Geometry: see drawing. Coordinates: mm, zero at the bounding-box minimum. A direction names the side the tool comes from. Give positions to 0.01 mm unless a question says otherwise; leave off trailing zeros. Order: outer loops, then holes, each group sorted by start corner. A loop starts at its lowest first (then second) coordinate and runs counter-clockwise, first axis right, second up. Notation, with made-up numbers: (39, -30) - (56, -30) arc R21 cw to (56, -21) - close; hole circle Ø8 at (55.5, 70.25). An arc over 180 degrees is marked (long way). Write each question's results on one line, items separated by ' | '. Start each with the question number.
Item 1: Contact query for a flat-ended pin moving along its axis: pin 1 Ø6 at (x, y) = (16.51, 56.34) entering from +Z. Output: stop coordinate, or through.
Item 2: Line query: line 1 along X through (y, z) = (55, 5.75); line 2 along Z through (x, y) = (3.5, 8). Output: solid intervals per line, ascending.
Item 3: Section C-C on y = 32.5. Output: boundary loops of the cut face in (x, z), and give its area (3 significant figures).
Item 4: Set-up query: the marked faces 1 and 2. Return all of +Z, -Z, +X, -X, +Y, -Y with unobstructed straight access to the full face (end or side cutting, diameter ignored); none if empty.
Item 5: Section A-A on z = 9.5. Output: boundary loops of the cut face in (x, y).
Item 6: Section B-B on y = 55. Output: boundary loops of the cut face in (x, z) (1 decimal).
Item 7: Section D-D on x = 10. Output: boundary loops of the cut face in (y, z).
Item 8: Mould query, pull axis X, two halves, no side actions, for the marked faces 3, 4 and 5. Classes: released by +X, released by -X, zero draft, split by the parting line, or undercut.
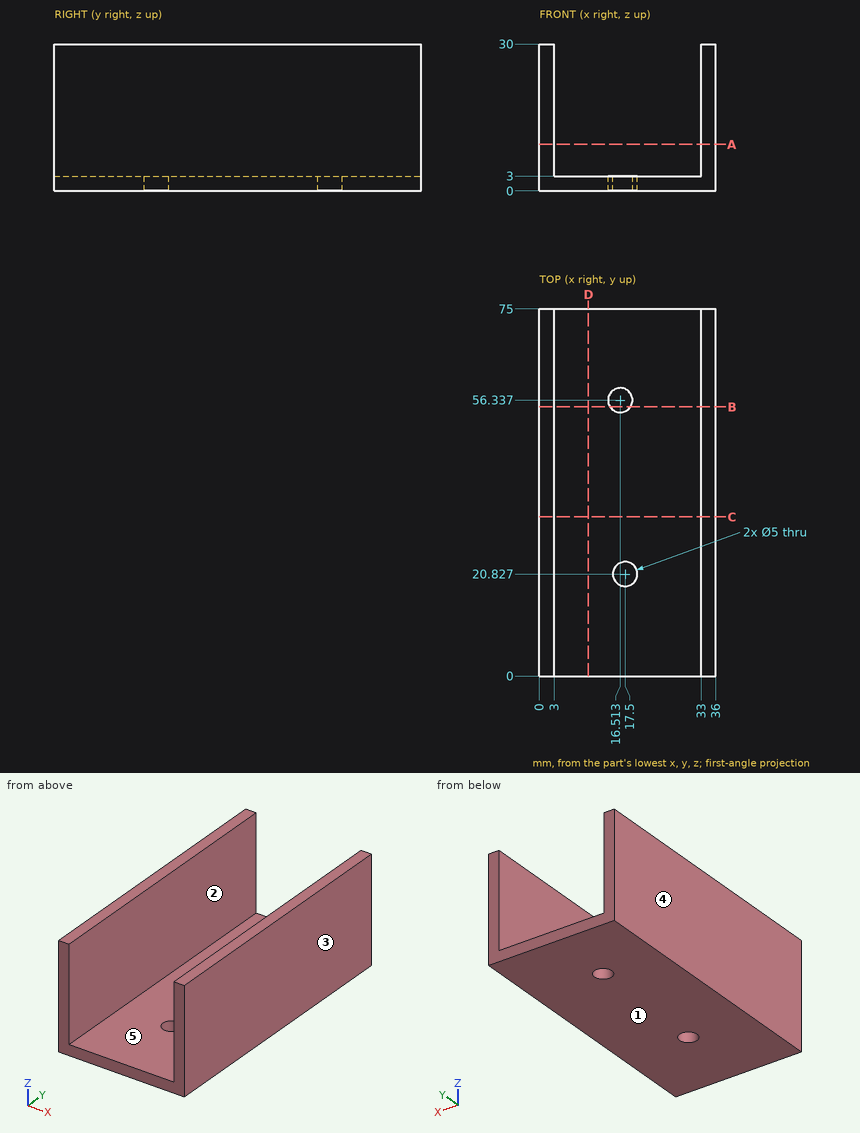
Evaluation:
1) pin 1: stops at z = 3
2) line 1: x = 0 to 3, 33 to 36 | line 2: z = 0 to 3
3) outline: (0, 0) - (36, 0) - (36, 30) - (33, 30) - (33, 3) - (3, 3) - (3, 30) - (0, 30) - close | area: 270 mm^2
4) face 1: -Z, +X, -X, +Y, -Y | face 2: +Z, +Y, -Y
5) outline: (0, 0) - (3, 0) - (3, 75) - (0, 75) - close; (33, 0) - (36, 0) - (36, 75) - (33, 75) - close
6) outline: (0, 0) - (14.4, 0) - (14.4, 3) - (3, 3) - (3, 30) - (0, 30) - close; (18.6, 0) - (36, 0) - (36, 30) - (33, 30) - (33, 3) - (18.6, 3) - close
7) outline: (0, 0) - (75, 0) - (75, 3) - (0, 3) - close
8) face 3: released by +X | face 4: released by -X | face 5: undercut
